Could you check a few things on this model? Use its own coordinates, in mm. A direction names the side the tool comes from. Coordinates: 2 decimals unless noted, no trailing zeros. Write each loop counter-clockwise with the first axis right and the second up, starting at its lowest first coordinate (ties: lowest second). Pieces come first, ordered by that corner, then holes. Notation, with made-up numbers: M -17,26.25 L -7,26.25 A25 cw -7,64.25 Z; hole C 34,78 d8. An arc over 180 degrees is marked long. Write item = value, one per line.
```python
from build123d import *

# Parameters (mm, degrees)
SKETCH1_R           = 5
BOSS_EXTRUDE1_DEPTH = 4
SKETCH1_3_R         = 5
SKETCH1_3_R_2       = 3
BOSS_EXTRUDE2_DEPTH = 8
SKETCH2_R           = 3
BOSS_EXTRUDE3_DEPTH = 4.5
CUT_EXTRUDE1_START  = -4.5
SKETCH3_R           = 3
CUT_EXTRUDE1_DEPTH  = 4.5
CHAMFER1_SIZE       = 1
FILLET1_R           = 1


with BuildPart() as part:
    # Sketch1 → Boss-Extrude1 (new body)
    with BuildSketch(Plane(origin=(0, 0, 0), x_dir=(1, 0, 0), z_dir=(0, 1, 0))):
        with BuildLine():
            Line((15, 4.5), (5.361902647, 4.5))
            ThreePointArc((5.361902647, 4.5), (-7, 0), (5.361902647, -4.5))
            Line((5.361902647, -4.5), (30, -4.5))
            Line((30, -4.5), (30, 0))
            Line((30, 0), (15, 0))
            Line((15, 0), (15, 4.5))
        make_face()
        with Locations(Location((0, 0, 0), (0, 0, 270))):
            Circle(SKETCH1_R, mode=Mode.SUBTRACT)
    extrude(amount=BOSS_EXTRUDE1_DEPTH)

    # Sketch1_3 → Boss-Extrude2 (add)
    with BuildSketch(Plane(origin=(0, 0, 0), x_dir=(1, 0, 0), z_dir=(0, 1, 0))):
        with Locations(Location((0, 0, 0), (0, 0, 270))):
            Circle(SKETCH1_3_R)
        with Locations(Location((0, 0, 0), (0, 0, 270))):
            Circle(SKETCH1_3_R_2, mode=Mode.SUBTRACT)
    extrude(amount=BOSS_EXTRUDE2_DEPTH)

    # Sketch2 → Boss-Extrude3 (add)
    with BuildSketch(Plane.XY):
        with BuildLine():
            Line((15, 4), (15, 0))
            Line((15, 0), (30, 0))
            Line((30, 0), (30, 4))
            ThreePointArc((30, 4), (22.5, 11.5), (15, 4))
        make_face()
        with Locations((22.5, 4)):
            Circle(SKETCH2_R, mode=Mode.SUBTRACT)
    extrude(amount=BOSS_EXTRUDE3_DEPTH)

    # Sketch3 → Cut-Extrude1 (cut)
    with BuildSketch(Plane.XY.offset(4.5).offset(CUT_EXTRUDE1_START)):
        with Locations((22.5, 4)):
            Circle(SKETCH3_R)
    extrude(amount=CUT_EXTRUDE1_DEPTH, mode=Mode.SUBTRACT)

    # Chamfer1
    chamfer1_edges = [part.edges().sort_by_distance(p)[0] for p in [
        (10.180951324, 4, -4.5),
        (10.180951324, 0, -4.5),
        (15, 2, -4.5),
        (10.180951324, 4, 4.5),
        (0, 4, -5),
        (30, 0, 2.25),
    ]]
    chamfer(chamfer1_edges, length=CHAMFER1_SIZE)

    # Fillet1
    fillet1_edges = [part.edges().sort_by_distance(p)[0] for p in [
        (15, 4, 1.75),
        (15.016722764, 3.499438512, 4.000561488),
    ]]
    fillet(fillet1_edges, radius=FILLET1_R)


solid = part.part
```
Item 1: Imagine slicing it at C-C (y = 1.5). Write out the boundary of the cut face in (x, z).
Numbers:
outline = M 5.36,-4.5 L 14,-4.5 L 15,-3.5 L 15,0 L 20.84,0 L 20.84,4.5 L 5.36,4.5 A7 ccw long Z; M 24.16,0 L 30,0 L 30,4.5 L 24.16,4.5 Z; hole C 0,0 d6
Item 2: Imagine slicing it at B-B (x = 0). Write out the boundary of the cut face in (y, z).
Numbers:
outline = M 0,-7 L 4,-7 L 4,-6 L 5,-5 L 8,-5 L 8,-3 L 0,-3 Z; M 0,3 L 8,3 L 8,5 L 5,5 L 4,6 L 4,7 L 0,7 Z
Item 3: Imagine slicing it at A-A (y = 6.5). Write out the boundary of the cut face in (x, z).
Numbers:
outline = C 0,0 d10; M 15.43,0 L 20.84,0 L 20.84,4.5 L 15.43,4.5 Z; M 24.16,0 L 29.57,0 L 29.57,4.5 L 24.16,4.5 Z; hole C 0,0 d6
Item 4: If I drill on line 1 along Y through (x, z) = (22.5, 3.55); line 2 along X through (y, z) = (2.25, 2.75); line 3 along Z through (x, y) = (22.5, 10.75), over which ranges is the centre line in solid material (lowest first)?
Numbers:
line_1 = 0 to 1, 7 to 11.5
line_2 = -6.44 to -1.2, 1.2 to 20.06, 24.94 to 30
line_3 = 0 to 4.5
Item 5: Imagine slicing it at D-D (z = 2). State how many separate pieces and enclosed holes the cut face has, and give its area (3 significant figures).
Numbers:
separate_pieces = 2
enclosed_holes = 1
area = 209 mm²
Item 6: For faces 4 (the face through (20, 7, 4.5)), 5 (the face through (15, 2, -2)), 6 (the face through (14.72, 4.25, 1.98)), 7 (the face through (10.2, 3.5, -4)), which set-ups out of +Z, -Z, +X, -X, +Y, -Y let a thin tool reach every point of the face, with its end or its side?
Numbers:
face_4 = +Z, +X, +Y, -Y
face_5 = -Z, +X, +Y, -Y
face_6 = +Z, -Z, +Y
face_7 = -Z, +X, +Y
Item 7: I'm going to push flat-ended pins straight in: P1, Ø6, axis at x = 13.5, y = 4, coming from the -Z side; P2, Ø4, axis at y = 1.5, z = 4, coming from the -X side; P3, Ø1, axis at y = 4, z = -5, coming from the +X side. Where does each tip first touch, or does it pass through?
Numbers:
P1 = -4.5
P2 = -6.71
P3 = 5.36
Item 8: If we mould it in two halves opening along X, with no side actions, what happens to faces 1 (the face through (14.6, 2, -3.9)), 2 (the face through (-3.3, 8, -0.1)), 3 (the face through (0.9, 3.94, 2.86))? For each: pulls with the +X half, pulls with the -X half, needs draft (parallel to the pull), parting line crosses it, or undercut.
Numbers:
face_1 = pulls with the +X half
face_2 = needs draft
face_3 = undercut
